from build123d import *

# Parameters (mm, degrees)
F0_W     = 50.8
F0_H     = 25.4
F0_W_2   = 47.625
F0_H_2   = 22.225
F1_DEPTH = 304.8
F2_R     = 14.28115
F3_DEPTH = 25.401
F4_R     = 14.2875
F4_R_2   = 2.5527
F5_DEPTH = 25.401
F7_D     = 5.1054
F9_D     = 5.1054


with BuildPart() as f1:
    # F0 (on Right) → F1 (new body)
    with BuildSketch(Plane.YZ):
        Rectangle(F0_W, F0_H)
        Rectangle(F0_W_2, F0_H_2, mode=Mode.SUBTRACT)
    extrude(amount=F1_DEPTH)

    # F2 (on face) → F3 (cut, through all)
    with BuildSketch(Plane.XY.offset(12.7)):
        with Locations((279.4, 0)):
            Circle(F2_R)
    extrude(amount=-F3_DEPTH, mode=Mode.SUBTRACT)

    # F4 (on face) → F5 (cut, through all)
    with BuildSketch(Plane.XY.offset(12.7)):
        with Locations((50.8, 0)):
            Circle(F4_R)
        with Locations((68.326, 17.526)):
            Circle(F4_R_2)
        with Locations((68.326, -17.526)):
            Circle(F4_R_2)
        with Locations((33.274, -17.526)):
            Circle(F4_R_2)
        with Locations((33.274, 17.526)):
            Circle(F4_R_2)
    extrude(amount=-F5_DEPTH, mode=Mode.SUBTRACT)

    # F7 (through all)
    with Locations(Plane.XZ.offset(25.4)):
        with Locations((165.1, 0), (139.7, 0), (63.5, 0), (114.3, 0), (266.7, 0), (88.9, 0), (12.7, 0), (190.5, 0), (241.3, 0), (215.9, 0), (292.1, 0), (38.1, 0)):
            Hole(F7_D / 2)

    # F9 (through all)
    with Locations(Plane.XY.offset(12.7)):
        with Locations((88.9, 12.7), (165.1, -12.7), (241.3, -12.7), (139.7, -12.7), (38.1, 12.7), (165.1, 12.7), (215.9, -12.7), (292.1, 12.7), (266.7, -12.7), (63.5, -12.7), (88.9, -12.7), (266.7, 12.7), (241.3, 12.7), (63.5, 12.7), (38.1, -12.7), (190.5, 12.7), (12.7, 12.7), (12.7, -12.7), (114.3, -12.7), (114.3, 12.7), (292.1, -12.7), (139.7, 12.7), (190.5, -12.7), (215.9, 12.7)):
            Hole(F9_D / 2)


solid = f1.part
The listing builds one solid part. Answer for the finished solid, in the listing's coordinates (mm). A direction names the side the tool comes from. Round coordinates to 2 decimals unless told otherwise and drop trailing zeros. Write each loop counter-clockwise with the first axis right and the second up, starting at its lowest first coordinate (ties: lowest second). Pieces come first, ordered by that corner, then holes. Notation, with made-up numbers: (54.25, -24) - (63.25, -24) arc R17 ccw to (63.25, -8) - close; hole circle Ø7 at (69.5, -28). An arc over 180 degrees is marked (long way). Use one line per item in the form item = value. Start each with the question number.
Item 1: A cutting plane is placed at D-D (z = -5.5). Write down the section's boundary in (x, y), plus the area to 3 significant figures.
Item 2: A cutting plane is placed at C-C (y = -2.5). Write down the section's boundary in (x, z).
Item 3: A tool of negligible diameter and unlimited length cuts with its end or side. For faces 1 (the flat face through (150, -23.812, 0)), 2 (the cylindrical face through (193.05, -12.59, -11.92)), from which of +Z, -Z, +X, -X, +Y, -Y can it reach the whole face along a straight path? Write none if from no direction.
Item 4: A cutting plane is placed at B-B (x = 50.8). Write down the section's boundary in (y, z), plus the area to 3 significant figures.
Item 5: Find the intervals of material crossed by line 1 (Y direction, x = 12.7, z = -11.7); line 2 (Y direction, x = 18.5, z = -5.5); line 3 (Y direction, x = 63.5, z = -12.05), in increasing order. Write a range as [from, to].
Item 6: A cutting plane is placed at A-A (x = 241.3). Give the number of separate pieces and of enclosed holes in the cut face, plus the area to 3 significant figures.
Item 7: Determine the mould class of faces 3 (the cylindrical face through (193.05, 24.62, 0.11)), 4 (the cylindrical face through (238.865, 13.467, -11.917)), 5 (the cylindrical face through (265.133, 0.628, 11.917)) for opening direction Y: +Y half, -Y half, draft (parallel to the pull), parting line (faces both ways), or undercut.
The answers:
q1.outline = (0, -25.4) - (304.8, -25.4) - (304.8, -23.81) - (0, -23.81) - close; (0, 23.81) - (304.8, 23.81) - (304.8, 25.4) - (0, 25.4) - close
q1.area = 968 mm^2
q2.outline = (0, -12.7) - (36.73, -12.7) - (36.73, -11.11) - (0, -11.11) - close; (0, 11.11) - (36.73, 11.11) - (36.73, 12.7) - (0, 12.7) - close; (64.87, -12.7) - (265.34, -12.7) - (265.34, -11.11) - (64.87, -11.11) - close; (64.87, 11.11) - (265.34, 11.11) - (265.34, 12.7) - (64.87, 12.7) - close; (293.46, -12.7) - (304.8, -12.7) - (304.8, -11.11) - (293.46, -11.11) - close; (293.46, 11.11) - (304.8, 11.11) - (304.8, 12.7) - (293.46, 12.7) - close
q3.face_1 = +X, -X
q3.face_2 = +Z, -Z
q4.outline = (-25.4, -12.7) - (-14.29, -12.7) - (-14.29, -11.11) - (-23.81, -11.11) - (-23.81, 11.11) - (-14.29, 11.11) - (-14.29, 12.7) - (-25.4, 12.7) - close; (14.29, -12.7) - (25.4, -12.7) - (25.4, 12.7) - (14.29, 12.7) - (14.29, 11.11) - (23.81, 11.11) - (23.81, -11.11) - (14.29, -11.11) - close
q4.area = 141 mm^2
q5.line_1 = [-25.4, -15.25], [-10.15, 10.15], [15.25, 25.4]
q5.line_2 = [-25.4, -23.81], [23.81, 25.4]
q5.line_3 = [-25.4, -15.25], [-10.15, -6.55], [6.55, 10.15], [15.25, 25.4]
q6.separate_pieces = 6
q6.enclosed_holes = 0
q6.area = 183 mm^2
q7.face_3 = draft
q7.face_4 = undercut
q7.face_5 = undercut
